Read the model definition and answer for the solid it produces. Units are mm, in the model's axes. A direction names the side the tool comes from. Coordinates: 2 decimals unless noted, no trailing zeros. Loops run counter-clockwise (first coordinate to the right, second up) from the corner with the lowest first, then second, coordinate; pieces in that order, holes last. Notation, with made-up numbers: (23.25, 62) -> (29.25, 62) arc R21 ccw to (29.25, 92) -> close; hole circle Ø6 at (75.25, -22.5). An arc over 180 degrees is marked (long way). Answer as a JSON object with one key per item and string values. Group by question number.
1) Which of the six approach directions +Z, -Z, +X, -X, +Y, -Y give full straight-line access (tool end or side, diameter ignored) to faces 1 (the face through (0, 2, 0)), 2 (the face through (4, 0, -2)), 3 (the face through (-1.952, 3.493, -0.434))?
2) Flat-ended cylindrical pins translate along their axes: P1, Ø1.5, axis at x = 3.5, y = 2, coming from the -Z side; P2, Ø1, axis at y = 3.5, z = 4, coming from the +X side; P3, Ø4, axis at x = -0.5, z = 1, coming from the -Y side. Find the tip coordinate at first contact, or state that the pin passes through.
3) Section A-A, the plane z = 0 is taken. Give the vertices of the cut face in (x, y).
4) Section C-C, the plane y = 1 is taken. Give the vertices of the cut face in (x, z), plus the area to 3 significant figures.
5) Section D-D, the plane y = 2.6 is taken. Give the vertices of the cut face in (x, z).
6) Consider probe 1 along X at (y, z) = (3.6, 0); probe 2 along X at (y, z) = (0.7, 0); probe 3 along Y at (x, z) = (1, 2.5). Determine where each line is inside the solid, lowest interval first. Write a range as [from, to].
7) Determine the mould class of faces 4 (the face through (-5.37, 1.97, -1.19)), 5 (the face through (-2.53, 0.99, -3.29)), 6 (the face through (-2.4, 4, -0.1)) for opening direction X: released by +X, released by -X, zero draft, split by the parting line, or undercut.
8) Section B-B, the plane x = 0 is taken. Give the vertices of the cut face in (y, z), plus the area to 3 significant figures.
from build123d import *

# Parameters (mm, degrees)
SKETCH1_R           = 5.5
SKETCH1_R_2         = 4.15
BOSS_EXTRUDE1_DEPTH = 3
SKETCH2_R           = 5.5
SKETCH2_R_2         = 2
BOSS_EXTRUDE2_DEPTH = 1
BOSS_EXTRUDE3_START = 1
SKETCH3_R           = 4.15
BOSS_EXTRUDE3_DEPTH = 1


with BuildPart() as part:
    # Sketch1 → Boss-Extrude1 (new body)
    with BuildSketch(Plane(origin=(0, 0, 0), x_dir=(1, 0, 0), z_dir=(0, 1, 0))):
        with Locations(Location((0, 0, 0), (0, 0, 270))):
            Circle(SKETCH1_R)
        with Locations(Location((0, 0, 0), (0, 0, 270))):
            Circle(SKETCH1_R_2, mode=Mode.SUBTRACT)
    extrude(amount=BOSS_EXTRUDE1_DEPTH)

    # Sketch2 → Boss-Extrude2 (add)
    with BuildSketch(Plane(origin=(0, 3, 0), x_dir=(1, 0, 0), z_dir=(0, 1, 0))):
        with Locations(Location((0, 0, 0), (0, 0, 270))):
            Circle(SKETCH2_R)
        with Locations(Location((0, 0, 0), (0, 0, 270))):
            Circle(SKETCH2_R_2, mode=Mode.SUBTRACT)
    extrude(amount=BOSS_EXTRUDE2_DEPTH)

    # Sketch3 → Boss-Extrude3 (add)
    with BuildSketch(Plane.XZ.offset(-3).offset(BOSS_EXTRUDE3_START)):
        with Locations(Location((0, 0, 0), (0, 0, 270))):
            Circle(SKETCH3_R)
    extrude(amount=-BOSS_EXTRUDE3_DEPTH)


solid = part.part
Determined:
{
 "1": {"face 1": "-Y", "face 2": "+Z, -Z, +X, -X, -Y", "face 3": "+Y"},
 "2": {"P1": "z = -4.76", "P2": "x = 4.24", "P3": "y = 2"},
 "3": {"outline": "(-5.5, 0) -> (-4.15, 0) -> (-4.15, 2) -> (4.15, 2) -> (4.15, 0) -> (5.5, 0) -> (5.5, 4) -> (2, 4) -> (2, 3) -> (-2, 3) -> (-2, 4) -> (-5.5, 4) -> close"},
 "4": {"outline": "circle Ø11 at (0, 0); hole circle Ø8.3 at (0, 0)", "area": "40.9 mm²"},
 "5": {"outline": "circle Ø11 at (0, 0)"},
 "6": {"probe 1": "[-5.5, -2], [2, 5.5]", "probe 2": "[-5.5, -4.15], [4.15, 5.5]", "probe 3": "[2, 4]"},
 "7": {"face 4": "split by the parting line", "face 5": "undercut", "face 6": "zero draft"},
 "8": {"outline": "(0, -5.5) -> (4, -5.5) -> (4, -2) -> (3, -2) -> (3, 2) -> (4, 2) -> (4, 5.5) -> (0, 5.5) -> (0, 4.15) -> (2, 4.15) -> (2, -4.15) -> (0, -4.15) -> close", "area": "23.4 mm²"}
}
